Could you check a few things on this model? Use its own coordinates, in mm. A direction names the side the tool comes from. Coordinates: 2 decimals unless noted, no trailing zeros. Loops run counter-clockwise (first coordinate to the right, second up) from the corner with the lowest first, then second, coordinate; pieces in that order, holes last. Notation, with made-up numbers: (-33, 81) - (-23, 81) arc R15 ccw to (-23, 101) - close; hole circle Ø9 at (35.5, -5). An arc over 180 degrees is marked (long way). One line per question, with ' | ' between items. Start each with the question number.
1. We'd pull the mould along Y, two halves only. Please class faces 3 (the flat face through (0, -2, 4.76)), 4 (the cylindrical face through (-22.587, 103.914, 24.87)): pulls with the +Y half, pulls with the -Y half, needs draft (parallel to the pull), parting line crosses it, or undercut.
2. Please list where these lines run through material, in increasing order: L1, parallel to X at y = 104, z = 29.5; L2, parallel to Z at x = -20, y = 102.5; L3, parallel to Y at x = -22.5, z = 24.76. Write a range as [from, to].
3. I want a section at B-B, the plane z = 24.76. Write out the boundary of the cut face in (x, y).
4. I want a section at C-C, the plane z = 35.5. Write out the boundary of the cut face in (x, y), then the cut area to 3 significant figures.
5. I want a section at D-D, the plane x = 18. Write out the boundary of the cut face in (y, z).
6. I'm going to push flat-ended pins straight in: P1, Ø1, axis at x = 17, z = 7, coming from the -Y side; P2, Ø4, axis at x = 14, y = -80.5, coming from the +Z side. Where does each tip first touch, or does it pass through?
7. Which directions (+Z, -Z, +X, -X, +Y, -Y) give clear straight access to the entire face, cutting with the end or side of a thin tool? Please do faces 1 (the flat face through (23, 2, 38)), 2 (the flat face through (-20.24, 2, 21)).
8. I want a section at A-A, the plane y = 52. Write out the boundary of the cut face in (x, z), then the cut area to 3 significant figures.
from build123d import *

# Parameters (mm, degrees)
F1_DEPTH      = 4.76
F4_DEPTH      = 38
F8_R          = 2.5
F9_DEPTH      = 4.7610001
F9_DEPTH_BACK = 45.2410001


# Not quite as in the source:
# - a feature names something its author has since deleted; it is built from what else it names


with BuildPart() as f1:
    # F0 (on Top) → F1 (new body)
    with BuildSketch(Plane.XY):
        with BuildLine():
            Line((20.24, 120.3093612318), (20.24, 123.3504860144))
            ThreePointArc((20.24, 123.3504860144), (10.1535522896, 124.5869390261), (0, 125))
            Line((0, 125), (0, 122))
            ThreePointArc((0, 122), (10.1552432202, 121.5766056244), (20.24, 120.3093612318))
        make_face()
        with BuildLine():
            Line((25, 90.3494910666), (25, 119.4110547646))
            ThreePointArc((25, 119.4110547646), (22.6244588582, 119.8838348626), (20.24, 120.3093612318))
            Line((20.24, 120.3093612318), (20.24, 105.3494910666))
            Line((20.24, 105.3494910666), (20.24, 90.3494910666))
            Line((20.24, 90.3494910666), (25, 90.3494910666))
        make_face()
        with BuildLine():
            ThreePointArc((-20.24, -120.3093612318), (-10.1552432202, -121.5766056244), (0, -122))
            Line((0, -122), (0, 0))
            Line((0, 0), (0, 101.8494910666))
            Line((0, 101.8494910666), (-3.5, 101.8494910666))
            Line((-3.5, 101.8494910666), (-3.5, 108.8494910666))
            Line((-3.5, 108.8494910666), (0, 108.8494910666))
            Line((0, 108.8494910666), (0, 122))
            ThreePointArc((0, 122), (-10.1552432202, 121.5766056244), (-20.24, 120.3093612318))
            Line((-20.24, 120.3093612318), (-20.24, 107.6747455333))
            Line((-20.24, 107.6747455333), (-20.24, 90.3494910666))
            Line((-20.24, 90.3494910666), (-20.24, -120.3093612318))
        make_face()
        with BuildLine():
            Line((0, 0), (0, -122))
            ThreePointArc((0, -122), (10.1552432202, -121.5766056244), (20.24, -120.3093612318))
            Line((20.24, -120.3093612318), (20.24, 90.3494910666))
            Line((20.24, 90.3494910666), (20.24, 105.3494910666))
            Line((20.24, 105.3494910666), (20.24, 120.3093612318))
            ThreePointArc((20.24, 120.3093612318), (10.1552432202, 121.5766056244), (0, 122))
            Line((0, 122), (0, 108.8494910666))
            Line((0, 108.8494910666), (3.5, 108.8494910666))
            Line((3.5, 108.8494910666), (3.5, 101.8494910666))
            Line((3.5, 101.8494910666), (0, 101.8494910666))
            Line((0, 101.8494910666), (0, 0))
        make_face()
        with BuildLine():
            Line((0, 122), (0, 125))
            ThreePointArc((0, 125), (-10.1535522896, 124.5869390261), (-20.24, 123.3504860144))
            Line((-20.24, 123.3504860144), (-20.24, 120.3093612318))
            ThreePointArc((-20.24, 120.3093612318), (-10.1552432202, 121.5766056244), (0, 122))
        make_face()
        with BuildLine():
            Line((25, -119.4110547646), (25, 90.3494910666))
            Line((25, 90.3494910666), (20.24, 90.3494910666))
            Line((20.24, 90.3494910666), (20.24, -120.3093612318))
            ThreePointArc((20.24, -120.3093612318), (22.6244588582, -119.8838348626), (25, -119.4110547646))
        make_face()
        with BuildLine():
            ThreePointArc((-20.24, 120.3093612318), (-22.6244588582, 119.8838348626), (-25, 119.4110547646))
            Line((-25, 119.4110547646), (-25, 90.3494910666))
            Line((-25, 90.3494910666), (-20.24, 90.3494910666))
            Line((-20.24, 90.3494910666), (-20.24, 107.6747455333))
            Line((-20.24, 107.6747455333), (-20.24, 120.3093612318))
        make_face()
        with BuildLine():
            ThreePointArc((-25, -119.4110547646), (-22.6244588582, -119.8838348626), (-20.24, -120.3093612318))
            Line((-20.24, -120.3093612318), (-20.24, 90.3494910666))
            Line((-20.24, 90.3494910666), (-25, 90.3494910666))
            Line((-25, 90.3494910666), (-25, -119.4110547646))
        make_face()
    extrude(amount=F1_DEPTH)

    # F0 (on Top) → F4 (join)
    with BuildSketch(Plane.XY):
        with BuildLine():
            ThreePointArc((-20.24, 123.3504860144), (-22.6242401752, 122.9355268281), (-25, 122.4744871392))
            Line((-25, 122.4744871392), (-25, 119.4110547646))
            ThreePointArc((-25, 119.4110547646), (-22.6244588582, 119.8838348626), (-20.24, 120.3093612318))
            Line((-20.24, 120.3093612318), (-20.24, 123.3504860144))
        make_face()
        with BuildLine():
            ThreePointArc((-20.24, 120.3093612318), (-22.6244588582, 119.8838348626), (-25, 119.4110547646))
            Line((-25, 119.4110547646), (-25, 90.3494910666))
            Line((-25, 90.3494910666), (-20.24, 90.3494910666))
            Line((-20.24, 90.3494910666), (-20.24, 107.6747455333))
            Line((-20.24, 107.6747455333), (-20.24, 120.3093612318))
        make_face()
        with BuildLine():
            Line((25, 90.3494910666), (25, 119.4110547646))
            ThreePointArc((25, 119.4110547646), (22.6244588582, 119.8838348626), (20.24, 120.3093612318))
            Line((20.24, 120.3093612318), (20.24, 105.3494910666))
            Line((20.24, 105.3494910666), (20.24, 90.3494910666))
            Line((20.24, 90.3494910666), (25, 90.3494910666))
        make_face()
        with BuildLine():
            Line((25, 119.4110547646), (25, 122.4744871392))
            ThreePointArc((25, 122.4744871392), (22.6242401752, 122.9355268281), (20.24, 123.3504860144))
            Line((20.24, 123.3504860144), (20.24, 120.3093612318))
            ThreePointArc((20.24, 120.3093612318), (22.6244588582, 119.8838348626), (25, 119.4110547646))
        make_face()
        with BuildLine():
            Line((25, -119.4110547646), (25, 90.3494910666))
            Line((25, 90.3494910666), (20.24, 90.3494910666))
            Line((20.24, 90.3494910666), (20.24, -120.3093612318))
            ThreePointArc((20.24, -120.3093612318), (22.6244588582, -119.8838348626), (25, -119.4110547646))
        make_face()
        with BuildLine():
            ThreePointArc((-25, -119.4110547646), (-22.6244588582, -119.8838348626), (-20.24, -120.3093612318))
            Line((-20.24, -120.3093612318), (-20.24, 90.3494910666))
            Line((-20.24, 90.3494910666), (-25, 90.3494910666))
            Line((-25, 90.3494910666), (-25, -119.4110547646))
        make_face()
    extrude(amount=F4_DEPTH)

    # F2 (on Front) → F6 (revolve, cut)
    with BuildSketch(Plane.XZ):
        with BuildLine():
            ThreePointArc((0, 128), (88.3883476483, 91.3883476483), (125, 3))
            Line((125, 3), (150, 3))
            ThreePointArc((150, 3), (106.066017178, 109.066017178), (0, 153))
            Line((0, 153), (0, 128))
        make_face()
    revolve(axis=Axis((0, 0, 64), (0, 0, 1)), mode=Mode.SUBTRACT)

    # F7: F1 across face


with BuildPart() as f1_1:
    add(f1.part)
    add(f1.part.mirror(Plane.XZ))

    # F8 (on face) → F9 (cut, two sides)
    with BuildSketch(Plane(origin=(20.24, 0, 0), x_dir=(0, -1, 0), z_dir=(-1, 0, 0))) as f9_sk:
        with Locations((-101.4159989458, 24.76)):
            Circle(F8_R)
    extrude(amount=-F9_DEPTH, mode=Mode.SUBTRACT)
    extrude(f9_sk.sketch, amount=F9_DEPTH_BACK, mode=Mode.SUBTRACT)


solid = f1_1.part
Results are:
1) face 3: needs draft | face 4: undercut
2) L1: x = [-25, -20.24], [20.24, 25] | L2: z = [0, 4.76] | L3: y = [-121.02, 98.92], [103.92, 121.02]
3) outline: (-25, -120.53) arc R123.09 ccw to (-20.24, -121.42) - (-20.24, 98.92) - (-25, 98.92) - close; (-25, 103.92) - (-20.24, 103.92) - (-20.24, 121.42) arc R123.09 ccw to (-25, 120.53) - close; (20.24, -121.42) arc R123.09 ccw to (25, -120.53) - (25, 98.92) - (20.24, 98.92) - close; (20.24, 103.92) - (25, 103.92) - (25, 120.53) arc R123.09 ccw to (20.24, 121.42) - close
4) outline: (-25, -118.08) arc R120.7 ccw to (-20.24, -118.99) - (-20.24, 118.99) arc R120.7 ccw to (-25, 118.08) - close; (20.24, -118.99) arc R120.7 ccw to (25, -118.08) - (25, 118.08) arc R120.7 ccw to (20.24, 118.99) - close | area: 2,260 mm2
5) outline: (-123.7, 0) - (123.7, 0) - (123.7, 3) arc R123.7 ccw to (123.68, 4.76) - (-123.68, 4.76) arc R123.7 ccw to (-123.7, 3) - close
6) P1: passes through | P2: stops at z = 4.76
7) face 1: +Z, +X, -X, +Y, -Y | face 2: +Z, +Y, -Y
8) outline: (-25, 0) - (25, 0) - (25, 38) - (20.24, 38) - (20.24, 4.76) - (-20.24, 4.76) - (-20.24, 38) - (-25, 38) - close | area: 554 mm2
